Here's how the part is built. I have some questions about the finished solid (model axes, mm). A direction names the side the tool comes from. Round coordinates to 2 decimals unless told otherwise and drop trailing zeros. Order: outer loops, then holes, each group sorted by start corner. A loop starts at its lowest first (then second) coordinate and runs counter-clockwise, first axis right, second up. Notation, with made-up numbers: (-28.5, 87) - (-7.5, 87) arc R14 cw to (-7.5, 101) - close; hole circle Ø5 at (-18.75, 62). An arc over 180 degrees is marked (long way). Answer as a JSON object with one key per item and string values.
```python
from build123d import *

# Parameters (mm, degrees)
PAD003_DEPTH    = 2.8
SKETCH_W        = 20
SKETCH_H        = 68
PAD_DEPTH       = 8
SKETCH276_W     = 20
SKETCH276_H     = 5
PAD001_DEPTH    = 5
SKETCH342_W     = 20
SKETCH342_H     = 29
PAD002_DEPTH    = 7.5
SKETCH343_R     = 1.8
POCKET_DEPTH    = 29.001
SKETCH347_W     = 20
SKETCH347_H     = 13
PAD004_DEPTH    = 5
SKETCH348_W     = 20
SKETCH348_H     = 8.4
POCKET001_DEPTH = 5
SKETCH345_R     = 4.2
POCKET002_DEPTH = 7
SKETCH346_R     = 4.5
POCKET003_DEPTH = 8.001
CHAMFER_SIZE    = 1
FILLET_R        = 2.9
FILLET001_R     = 1.5


with BuildPart() as pad003:
    # Sketch344 → Pad003 (new body)
    with BuildSketch(Plane.XY.offset(23)):
        Polygon((-8.4, 25), (-2.6, 25), (-2.6, 35), (-5.5, 38), (-8.4, 35), align=None)
        Polygon((2.6, 25), (8.4, 25), (8.4, 35), (5.5, 38), (2.6, 35), align=None)
    extrude(amount=-PAD003_DEPTH)


with BuildPart() as fillet001:
    # Sketch → Pad (new body)
    with BuildSketch(Plane.XY):
        Rectangle(SKETCH_W, SKETCH_H)
    extrude(amount=PAD_DEPTH)

    # Sketch276 → Pad001 (new body)
    with BuildSketch(Plane.XY.offset(8)):
        with Locations((0, -23.5)):
            Rectangle(SKETCH276_W, SKETCH276_H)
    extrude(amount=PAD001_DEPTH)

    # Sketch342 → Pad002 (new body, symmetric)
    with BuildSketch(Plane(origin=(0, 34, 0), x_dir=(-1, 0, 0), z_dir=(0, 1, 0))):
        with Locations((0, 14.5)):
            Rectangle(SKETCH342_W, SKETCH342_H)
    extrude(amount=PAD002_DEPTH, both=True)

    # Sketch343 → Pocket (cut, through all)
    with BuildSketch(Plane.XY.offset(29)):
        with Locations((-5.5, 34)):
            Circle(SKETCH343_R)
        with Locations((5.5, 34)):
            Circle(SKETCH343_R)
    extrude(amount=-POCKET_DEPTH, mode=Mode.SUBTRACT)

    # Cut: cut Pad003
    add(pad003.part, mode=Mode.SUBTRACT)

    # Sketch347 → Pad004 (new body)
    with BuildSketch(Plane.XZ.offset(34)):
        with Locations((0, 6.5)):
            Rectangle(SKETCH347_W, SKETCH347_H)
    extrude(amount=PAD004_DEPTH)

    # Sketch348 → Pocket001 (cut)
    with BuildSketch(Plane.XY.offset(13)):
        with Locations((0, -30)):
            Rectangle(SKETCH348_W, SKETCH348_H)
    extrude(amount=-POCKET001_DEPTH, mode=Mode.SUBTRACT)

    # Sketch345 → Pocket002 (cut)
    with BuildSketch(Plane.XY.offset(13)):
        with Locations((-5, -30)):
            Circle(SKETCH345_R)
        with Locations((5, -30)):
            Circle(SKETCH345_R)
    extrude(amount=-POCKET002_DEPTH, mode=Mode.SUBTRACT)

    # Sketch346 → Pocket003 (cut, through all)
    with BuildSketch(Plane.XY.offset(8)):
        with Locations((0, 19)):
            Circle(SKETCH346_R)
    extrude(amount=-POCKET003_DEPTH, mode=Mode.SUBTRACT)

    # Chamfer
    chamfer_edges = [fillet001.edges().sort_by_distance(p)[0] for p in [
        (0, -25.8, 13),
        (0, -34.2, 13),
    ]]
    chamfer(chamfer_edges, length=CHAMFER_SIZE)

    # Fillet
    fillet_edges = [fillet001.edges().sort_by_distance(p)[0] for p in [
        (0, 26.5, 8),
        (0, 41.5, 0),
        (0, -39, 0),
        (0, -21, 8),
    ]]
    fillet(fillet_edges, radius=FILLET_R)

    # Fillet001
    fillet001_edges = [fillet001.edges().sort_by_distance(p)[0] for p in [
        (0, -39, 13),
        (-10, -39, 7.95),
        (10, -39, 7.95),
        (0, -21, 13),
        (-10, 1.25, 0),
        (-10, 41.5, 15.95),
        (-10, 26.5, 19.95),
        (-10, 2.75, 8),
        (10, 2.75, 8),
        (0, 26.5, 29),
        (-10, 34, 29),
        (0, 41.5, 29),
        (10, 41.5, 15.95),
        (10, 34, 29),
        (10, 1.25, 0),
    ]]
    fillet(fillet001_edges, radius=FILLET001_R)


solid = fillet001.part
```
1. For faces 1 (the face through (4.07, 36.52, 21.62)), 2 (the face through (10, 10, 6)), 3 (the face through (5.266, 35.785, 26.042)), 4 (the face through (0, -36, 13)), 5 (the face through (-9.4, -30, 8)), which set-ups out of +Z, -Z, +X, -X, +Y, -Y let a thin tool reach every point of the face, with its end or its side?
Responses:
{"face 1": "-Y", "face 2": "+Z, -Z, +X, +Y, -Y", "face 3": "+Z, -Z", "face 4": "+Z, +X, -X, -Y", "face 5": "+Z, +X, -X"}
2. Imagine slicing it at A-A (x = 0). List the corners of the cut face in (y, z) for me.
Responses:
{"outline": "(-39, 2.9) arc R2.9 ccw to (-36.1, 0) - (14.5, 0) - (14.5, 8) - (-18.1, 8) arc R2.9 cw to (-21, 10.9) - (-21, 11.5) arc R1.5 ccw to (-22.5, 13) - (-24.8, 13) - (-25.8, 12) - (-25.8, 8) - (-34.2, 8) - (-34.2, 12) - (-35.2, 13) - (-37.5, 13) arc R1.5 ccw to (-39, 11.5) - close; (23.5, 0) - (38.6, 0) arc R2.9 ccw to (41.5, 2.9) - (41.5, 27.5) arc R1.5 ccw to (40, 29) - (28, 29) arc R1.5 ccw to (26.5, 27.5) - (26.5, 10.9) arc R2.9 cw to (23.6, 8) - (23.5, 8) - close"}
3. Thinking about a two-plate mould opening in Y: for faces 6 (the face through (5, 31, 23)), 7 (the face through (-0.12, 41.07, 28.55)), 8 (the face through (-6.93, 36.52, 21.62)), 9 (the face through (0, -30, 8)), which applies, pulls with the +Y half, pulls with the -Y half, needs draft (parallel to the pull), parting line crosses it, or undercut?
Responses:
{"face 6": "needs draft", "face 7": "pulls with the +Y half", "face 8": "pulls with the -Y half", "face 9": "undercut"}
4. For P1, Ø5, axis at x = -4, z = 25.5, coming from the -Y side; P2, Ø6.5, axis at x = -6, y = -29.5, coming from the +Z side; P3, Ø9, axis at x = 6, y = -30, coming from the +Z side, each with a flat end and sliding along its axis, tell me the tip position at first contact or that it passes through.
Responses:
{"P1": "y = 26.5", "P2": "z = 8", "P3": "z = 12.3"}
5. If I drill on L1, parallel to X at y = -30, z = 7.05; L2, parallel to Y at x = -5.5, z = 26.5; L3, parallel to Y at x = 0, z = 5.75, over which ranges is the centre line in solid material (lowest first)? Write a range as [from, to].
Responses:
{"L1": "[-10, -9.2], [-0.8, 0.8], [9.2, 10]", "L2": "[26.5, 32.2], [35.8, 41.5]", "L3": "[-39, 14.5], [23.5, 41.5]"}
6. Imagine slicing it at D-D (y = -10.5). List the corners of the cut face in (x, z) for me, plus the area to 3 significant figures.
Responses:
{"outline": "(-10, 1.5) arc R1.5 ccw to (-8.5, 0) - (8.5, 0) arc R1.5 ccw to (10, 1.5) - (10, 6.5) arc R1.5 ccw to (8.5, 8) - (-8.5, 8) arc R1.5 ccw to (-10, 6.5) - close", "area": "158 mm2"}
7. Imagine slicing it at C-C (z = 23.75). List the corners of the cut face in (x, y) for me.
Responses:
{"outline": "(-10, 28) arc R1.5 ccw to (-8.5, 26.5) - (8.5, 26.5) arc R1.5 ccw to (10, 28) - (10, 40) arc R1.5 ccw to (8.5, 41.5) - (-8.5, 41.5) arc R1.5 ccw to (-10, 40) - close; hole circle Ø3.6 at (-5.5, 34); hole circle Ø3.6 at (5.5, 34)"}
8. Imagine slicing it at B-B (y = 19). List the corners of the cut face in (x, z) for me.
Responses:
{"outline": "(-10, 1.5) arc R1.5 ccw to (-8.5, 0) - (-4.5, 0) - (-4.5, 8) - (-8.5, 8) arc R1.5 ccw to (-10, 6.5) - close; (4.5, 0) - (8.5, 0) arc R1.5 ccw to (10, 1.5) - (10, 6.5) arc R1.5 ccw to (8.5, 8) - (4.5, 8) - close"}
